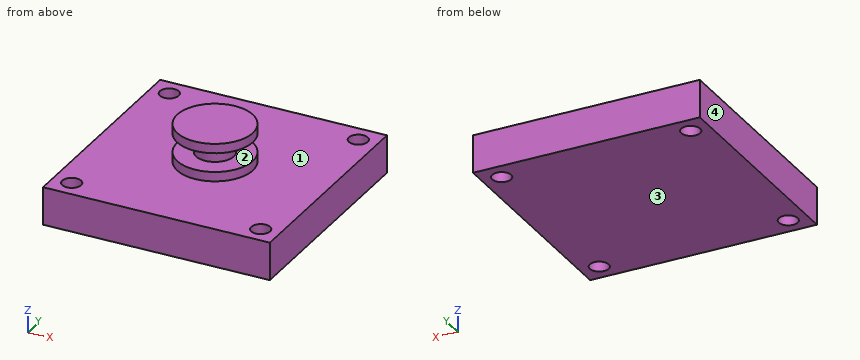
```python
from build123d import *

# Parameters (mm, degrees)
F0_W     = 152.4
F0_H     = 152.4
F1_DEPTH = 25.4
F2_R     = 6.35
F3_DEPTH = 25.401
F4_W     = 25.4
F4_H     = 25.4
F6_W     = 25.4
F6_H     = 12.7


with BuildPart() as f1:
    # F0 (on Top) → F1 (new body)
    with BuildSketch(Plane.XY):
        Rectangle(F0_W, F0_H)
    extrude(amount=F1_DEPTH)

    # F2 (on face) → F3 (cut, through all)
    with BuildSketch(Plane.XY.offset(25.4)):
        with Locations((-63.5, 63.5)):
            Circle(F2_R)
        with Locations((63.5, 63.5)):
            Circle(F2_R)
        with Locations((63.5, -63.5)):
            Circle(F2_R)
        with Locations((-63.5, -63.5)):
            Circle(F2_R)
    extrude(amount=-F3_DEPTH, mode=Mode.SUBTRACT)

    # F4 (on Front) → F5 (revolve)
    with BuildSketch(Plane.XZ):
        with Locations((-12.7, 38.1)):
            Rectangle(F4_W, F4_H)
    revolve(axis=Axis((0, 0, 38.1), (0, 0, 1)))

    # F6 (on Front) → F7 (revolve, cut)
    with BuildSketch(Plane.XZ):
        with Locations((-25.4, 38.1)):
            Rectangle(F6_W, F6_H)
    revolve(axis=Axis((0, 0, 50.8), (0, 0, -1)), mode=Mode.SUBTRACT)


solid = f1.part
```
Can you work these out from the model? Positions are in its coordinate system, mm. Face numbers are marked on the shaded views. Round coordinates to 2 decimals unless told otherwise and drop trailing zeros. Order: outer loops, then holes, each group sorted by start corner. A loop starts at its lowest first (then second) coordinate and runs counter-clockwise, first axis right, second up.
(1) If we section it at D-D (y = 0): Please give me the cut outline in (x, z).
Results are:
outline: (-76.2, 0) - (76.2, 0) - (76.2, 25.4) - (25.4, 25.4) - (25.4, 31.75) - (12.7, 31.75) - (12.7, 44.45) - (25.4, 44.45) - (25.4, 50.8) - (-25.4, 50.8) - (-25.4, 44.45) - (-12.7, 44.45) - (-12.7, 31.75) - (-25.4, 31.75) - (-25.4, 25.4) - (-76.2, 25.4) - close
(2) I'm going to push flat-ended pins straight in: pin 1 (2 mm diameter, centred on x = -11, z = 43, fed in from +Y); pin 2 (14.5 mm diameter, centred on x = -63.5, y = -63.5, fed in from +Z); pin 3 (6 mm diameter, centred on y = -3, z = 28.5, fed in from -X). Where does each tip first touch, or does it pass through?
Results are:
pin 1: stops at y = 7.83
pin 2: stops at z = 25.4
pin 3: stops at x = -25.4
(3) If we section it at C-C (z = 8.5): Please give me the cut outline in (x, y).
Results are:
outline: (-76.2, -76.2) - (76.2, -76.2) - (76.2, 76.2) - (-76.2, 76.2) - close; hole circle Ø12.7 at (-63.5, -63.5); hole circle Ø12.7 at (-63.5, 63.5); hole circle Ø12.7 at (63.5, -63.5); hole circle Ø12.7 at (63.5, 63.5)
(4) If I drill on L1, parallel to X at y = 63, z = 11; L2, parallel to Z at x = 0, y = -13.5; L3, parallel to Z at x = 39.5, y = 60, over which ranges is the centre line in solid material (lowest first)?
Results are:
L1: x = -76.2 to -69.83, -57.17 to 57.17, 69.83 to 76.2
L2: z = 0 to 31.75, 44.45 to 50.8
L3: z = 0 to 25.4
(5) If we section it at A-A (y = 63.5): Please give me the cut outline in (x, z).
Results are:
outline: (-76.2, 0) - (-69.85, 0) - (-69.85, 25.4) - (-76.2, 25.4) - close; (-57.15, 0) - (57.15, 0) - (57.15, 25.4) - (-57.15, 25.4) - close; (69.85, 0) - (76.2, 0) - (76.2, 25.4) - (69.85, 25.4) - close
(6) We'd pull the mould along Z, two halves only. Please class the marked faces 1, 2, 3 and 4: +Z half, -Z half, draft (parallel to the pull), parting line (faces both ways), or undercut.
Results are:
face 1: +Z half
face 2: undercut
face 3: -Z half
face 4: draft
